Drawing for the job (mm, zero at the part's lowest x, y, z). Round coordinates to 2 decimals unless told otherwise and drop trailing zeros. Write each loop counter-clockwise with the first axis right and the second up, starting at its lowest first coordinate (ties: lowest second). Pieces come first, ordered by that corner, then holes.
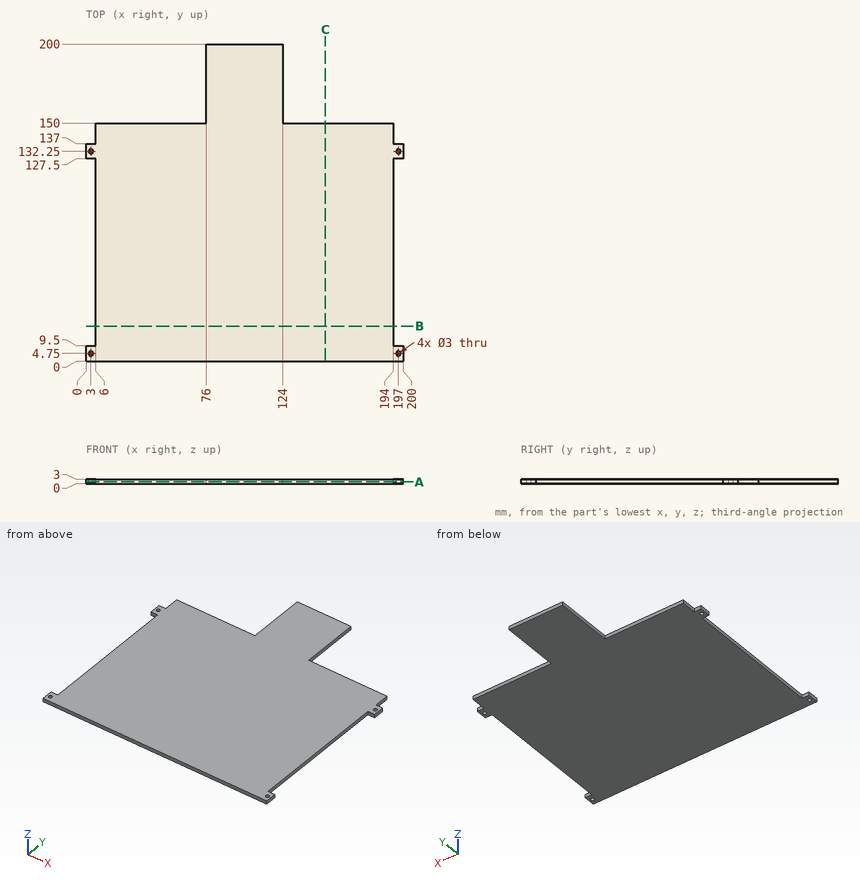
Q1. Saw through at C-C, the plane x = 151. Write the cut outline in (y, z).
Q2. Wall check: line 1 (X direction, y = 4.75, z = 0.8); line 2 (Y direction, x = 197, z = 1); line 3 (X direction, y = 143, z = 0.45). Give the ranges that are in metal, low to high.
Q3. Saw through at B-B, the plane y = 22. Write the cut outline in (x, z), and give its area (3 significant figures).
Q4. Saw through at A-A, the plane z = 1.25. Write the cut outline in (x, y).
Q5. Drop flat-ended pins along their axis: P1, Ø0.9, axis at x = 24, z = 2, coming from the +Y side; P2, Ø1.8, axis at x = 3, y = 4.75, coming from the -Z side; P3, Ø0.9, axis at y = 179, z = 1.5, coming from the +X side. Give the stop position or say it passes through.
Computed:
1. outline: (0, 0) - (150, 0) - (150, 3) - (0, 3) - close
2. line 1: x = 0 to 1.5, 4.5 to 195.5, 198.5 to 200
2. line 2: y = 0 to 3.25, 6.25 to 9.5, 127.5 to 130.75, 133.75 to 137
2. line 3: x = 6 to 194
3. outline: (6, 0) - (194, 0) - (194, 3) - (6, 3) - close
3. area: 564 mm2
4. outline: (0, 0) - (200, 0) - (200, 9.5) - (194, 9.5) - (194, 127.5) - (200, 127.5) - (200, 137) - (194, 137) - (194, 150) - (124, 150) - (124, 200) - (76, 200) - (76, 150) - (6, 150) - (6, 137) - (0, 137) - (0, 127.5) - (6, 127.5) - (6, 9.5) - (0, 9.5) - close; hole circle Ø3 at (3, 4.75); hole circle Ø3 at (3, 132.25); hole circle Ø3 at (197, 4.75); hole circle Ø3 at (197, 132.25)
5. P1: stops at y = 150
5. P2: passes through
5. P3: stops at x = 124
